Autodesk Inventor part; units mm, degrees
ref_plane "YZ Plane" through (0, 0, 0) normal (1, 0, 0) x (0, 1, 0)
ref_plane "XY Plane" through (0, 0, 0) normal (0, 0, 1) x (1, 0, 0)
sketch "Sketch1" plane through (0, 0, 0) normal (0, 1, 0) x (-1, 0, 0)
  line L0 (11.43, 11.43) -> (-11.43, 11.43)
  line L1 (-11.43, 11.43) -> (-11.43, -11.43)
  line L2 (-11.43, -11.43) -> (11.43, -11.43)
  line L3 (11.43, -11.43) -> (11.43, 11.43)
  line L4 (0.381, -11.43) -> (0.381, 11.43)
  line L5 (-0.381, -11.43) -> (-0.381, 11.43)
  line L6 (11.43, -0.381) -> (-11.43, -0.381)
  line L7 (11.43, 0.381) -> (-11.43, 0.381)
  circle A0 centre (0, 0) radius 5.08
  line L8 (12.446, -12.446) -> (-12.446, -12.446)
  line L9 (-12.446, -12.446) -> (-12.446, 12.446)
  line L10 (-12.446, 12.446) -> (12.446, 12.446)
  line L11 (12.446, 12.446) -> (12.446, -12.446)
  dimension "d0" = 22.86
  dimension "d1" = 22.86
  dimension "d2" = 11.43
  dimension "d3" = 11.43
  dimension "d7" = 0.381
  dimension "d8" = 0.762
  dimension "d12" = 0.381
  dimension "d13" = 0.381
  dimension "d14" = 0.762
  dimension "d21" = 10.16
  dimension "d28" = 1.016
  dimension "d29" = 1.016
  dimension "d30" = 1.016
  dimension "d31" = 1.016
extrude "Extrusion2" add sketch "Sketch1" against normal blind 22.86 contours L3 L7 A0 L4 L0 | L4 A0 L5 L0 | L3 L6 A0 L7 | L5 A0 L7 L1 L0 | A0 L7 L4 | L4 L7 L5 A0 | L3 L2 L4 A0 L6 | A0 L6 L4 L7 | L5 L7 A0 | L4 L6 L5 L7 | A0 L4 L6 | L7 A0 L6 L1 | L5 L6 A0 L7 | L4 A0 L5 L6 | L2 L5 A0 L4 | L6 A0 L5 L2 L1 | L5 A0 L6
extrude "Extrusion3" cut sketch "Sketch1" against normal blind 0.254 contours L4 A0 L5 L0 | L3 L6 A0 L7 | L4 L7 L5 A0 | A0 L6 L4 L7 | L4 L6 L5 L7 | L7 A0 L6 L1 | L5 L6 A0 L7 | L4 A0 L5 L6 | L2 L5 A0 L4
extrude "Extrusion4" add sketch "Sketch1" along normal blind 0.508 contours A0 L7 L4 | L4 L7 L5 A0 | A0 L6 L4 L7 | L5 L7 A0 | L4 L6 L5 L7 | A0 L4 L6 | L5 L6 A0 L7 | L4 A0 L5 L6 | L5 A0 L6
sketch "Sketch3" plane through (0, 0, 0) normal (0, 1, 0) x (-1, 0, 0)
  line L0 (11.43, -11.43) -> (11.43, -0.381)
  line L1 (-11.43, 11.43) -> (-11.43, 0.381)
  line L2 (11.43, -11.43) -> (-11.43, -11.43)
  line L3 (-11.43, -11.43) -> (-11.43, 11.43)
  line L4 (-11.43, 11.43) -> (11.43, 11.43)
  line L5 (11.43, 11.43) -> (11.43, -11.43)
  point P0 (0, 0)
extrude "Extrusion5" add sketch "Sketch3" along normal blind 3.175
sketch "Sketch4" plane through (0, 0, 0) normal (0, 1, 0) x (-1, 0, 0)
  circle A0 centre (0, -0.381) radius 8.0989
  point P0 (0, 0)
properties part number "companion_cube"
Input: part model. Units: mm. Frame: model coordinates. A direction names the side the tool comes from. Round coordinates to 2 decimals unless told otherwise and drop trailing zeros. One line per question, with ' | ' between items. Start each with the question number.
1) Pull-direction query (Z, two-part tool) for faces 3 (the flat face through (0, 0, 0)), 4 (the flat face through (0, -10, -11.43)), 5 (the flat face through (-11.43, -10, 0)); classes: +Z half, -Z half, draft (parallel to the pull), parting line (faces both ways), or undercut.
2) Set-up query: faces 1 (the flat face through (0, -10, 11.43)), 2 (the flat face through (0, -0.254, 0)). Return all of +Z, -Z, +X, -X, +Y, -Y with unobstructed straight access to the full face (end or side cutting, diameter ignored); none if empty.
3) Ray query, probe 1 along Y at (x, z) = (7.25, 0) (3 decimals). Return the intervals inside material, ascending.
Worked out:
1) face 3: undercut | face 4: -Z half | face 5: draft
2) face 1: +Z, +X, -X, +Y, -Y | face 2: none
3) probe 1: y = -22.86 to -0.254, 0 to 3.175
